Check sheet for the modelled part. Datum: model origin and axes. Units: mm. A direction names the side the tool comes from. Round coordinates to 2 decimals unless told otherwise and drop trailing zeros. Write each loop counter-clockwise with the first axis right and the second up, starting at its lowest first coordinate (ties: lowest second). Pieces come first, ordered by that corner, then holes.
Item 1: Tool access check on faces 5 (the flat face through (16, 0, -16)), 6 (the flat face through (8.58, 11.75, -8.78)). Record the directions out of +Z, -Z, +X, -X, +Y, -Y that give a thin tool (end or side, any length) a straight path to the whole face; none if there is none.
Item 2: Material ranges on line 1 (Y direction, x = 8.5, z = -17), recorded low to high.
Item 3: Cross-section at B-B on x = 13. Enter the section's corners in (y, z), plus the area to 3 significant figures.
Item 4: Cross-section at A-A on z = -16.5. Enter the section's corners in (x, y), plus the area to 3 significant figures.
Item 5: Release check for a two-part mould opening along Z. For faces 1 (the flat face through (22.72, 11.75, -8.58)), 2 (the flat face through (31.5, 6, -16)), 3 (the flat face through (16, 6, 0)), 4 (the flat face through (22.92, 11.75, -22.72)) record: +Z half, -Z half, draft (parallel to the pull), parting line (faces both ways), or undercut.
from build123d import *

# Parameters (mm, degrees)
SKETCH1_W           = 31.5
SKETCH1_H           = 31.5
BOSS_EXTRUDE1_DEPTH = 12
CUT_EXTRUDE1_DEPTH  = 0.5


with BuildPart() as part:
    # Sketch1 → Boss-Extrude1 (new body)
    with BuildSketch(Plane(origin=(0, 0, 0), x_dir=(1, 0, 0), z_dir=(0, 1, 0))):
        with Locations((15.75, 15.75)):
            Rectangle(SKETCH1_W, SKETCH1_H)
    extrude(amount=BOSS_EXTRUDE1_DEPTH)

    # Sketch3 → Cut-Extrude1 (cut)
    with BuildSketch(Plane(origin=(0, 12, 0), x_dir=(1, 0, 0), z_dir=(0, 1, 0))):
        Polygon((1.607864376, 15.75), (15.75, 1.607864376), (29.892135624, 15.75), (15.75, 29.892135624), align=None)
    extrude(amount=-CUT_EXTRUDE1_DEPTH, mode=Mode.SUBTRACT)


solid = part.part
Response values:
1. face 5: +Z, -Z, +X, -X, -Y
1. face 6: +Y
2. line 1: y = 0 to 11.5
3. outline: (0, -31.5) - (12, -31.5) - (12, -27.14) - (11.5, -27.14) - (11.5, -4.36) - (12, -4.36) - (12, 0) - (0, 0) - close
3. area: 367 mm2
4. outline: (0, 0) - (31.5, 0) - (31.5, 12) - (29.14, 12) - (29.14, 11.5) - (2.36, 11.5) - (2.36, 12) - (0, 12) - close
4. area: 365 mm2
5. face 1: undercut
5. face 2: draft
5. face 3: +Z half
5. face 4: undercut
